Here's how the part is built. I have some questions about the finished solid (model axes, mm). A direction names the side the tool comes from. Coordinates: 2 decimals unless noted, no trailing zeros. Write each loop counter-clockwise with the first axis right and the second up, starting at its lowest first coordinate (ties: lowest second). Pieces come first, ordered by that corner, then holes. Notation, with made-up numbers: M -23,-0.5 L 19,-0.5 A12 ccw 19,17.5 Z; hole C -26.5,14 d8. An arc over 180 degrees is marked long. Use a Markdown table: item, result.
```python
from build123d import *

# Parameters (mm, degrees)
SKETCH1_W           = 60.96
SKETCH1_H           = 40.64
BOSS_EXTRUDE1_DEPTH = 17.78
SHELL1_T            = -2.54
SKETCH2_R           = 2.54
BOSS_EXTRUDE2_DEPTH = 17.78
SKETCH3_R           = 1.016
CUT_EXTRUDE2_DEPTH  = 7.62
SKETCH5_W           = 7.62
SKETCH5_H           = 3.81
CUT_EXTRUDE3_DEPTH  = 2.54
FILLET1_R           = 1.27
SKETCH6_W           = 40.64
SKETCH6_H           = 19.05
CUT_EXTRUDE4_DEPTH  = 2.54
FILLET3_R           = 2.54


with BuildPart() as part:
    # Sketch1 → Boss-Extrude1 (new body)
    with BuildSketch(Plane(origin=(0, 0, 0), x_dir=(1, 0, 0), z_dir=(0, 1, 0))):
        with Locations((30.48, 20.32)):
            Rectangle(SKETCH1_W, SKETCH1_H)
    extrude(amount=BOSS_EXTRUDE1_DEPTH)

    # Shell1
    shell1_openings = [part.faces().sort_by_distance(p)[0] for p in [
        (30.48, 17.78, -20.32),
    ]]
    offset(amount=SHELL1_T, openings=shell1_openings, kind=Kind.INTERSECTION)

    # Sketch2 → Boss-Extrude2 (add)
    with BuildSketch(Plane(origin=(0, 17.78, 0), x_dir=(1, 0, 0), z_dir=(0, 1, 0))):
        with Locations((2.54, 2.54)):
            Circle(SKETCH2_R)
        with Locations((58.42, 2.54)):
            Circle(SKETCH2_R)
        with Locations((58.42, 38.1)):
            Circle(SKETCH2_R)
        with Locations((2.54, 38.1)):
            Circle(SKETCH2_R)
    extrude(amount=-BOSS_EXTRUDE2_DEPTH)

    # Sketch3 → Cut-Extrude2 (cut)
    with BuildSketch(Plane(origin=(0, 17.78, 0), x_dir=(1, 0, 0), z_dir=(0, 1, 0))):
        with Locations(Location((2.525101816, 38.1, 0), (0, 0, 270))):
            Circle(SKETCH3_R)
        with Locations(Location((2.525101816, 2.54, 0), (0, 0, 270))):
            Circle(SKETCH3_R)
        with Locations(Location((58.42, 2.54, 0), (0, 0, 270))):
            Circle(SKETCH3_R)
        with Locations(Location((58.42, 38.1, 0), (0, 0, 270))):
            Circle(SKETCH3_R)
    extrude(amount=-CUT_EXTRUDE2_DEPTH, mode=Mode.SUBTRACT)

    # Sketch5 → Cut-Extrude3 (cut)
    with BuildSketch(Plane(origin=(60.96, 0, 0), x_dir=(0, 0, -1), z_dir=(1, 0, 0))):
        with Locations((15.24, 15.875)):
            Rectangle(SKETCH5_W, SKETCH5_H)
    extrude(amount=-CUT_EXTRUDE3_DEPTH, mode=Mode.SUBTRACT)

    # Fillet1
    fillet1_edges = [part.edges().sort_by_distance(p)[0] for p in [
        (59.69, 13.97, -19.05),
        (59.69, 13.97, -11.43),
    ]]
    fillet(fillet1_edges, radius=FILLET1_R)

    # Sketch6 → Cut-Extrude4 (cut)
    with BuildSketch(Plane.XZ):
        with Locations((35.56, -28.575)):
            Rectangle(SKETCH6_W, SKETCH6_H)
    extrude(amount=-CUT_EXTRUDE4_DEPTH, mode=Mode.SUBTRACT)

    # Fillet3
    fillet3_edges = [part.edges().sort_by_distance(p)[0] for p in [
        (30.48, 0, -40.64),
        (60.96, 0, -20.32),
        (30.48, 0, 0),
        (0, 0, -20.32),
        (0, 8.89, -40.64),
        (60.96, 8.89, -40.64),
        (60.96, 8.89, 0),
        (0, 8.89, 0),
    ]]
    fillet(fillet3_edges, radius=FILLET3_R - 0.0001)  # a hair under: the kernel refuses the full size


solid = part.part
```
1. Suppose I cut it at B-B on z = -31.5. Write out the boundary of the cut face in (x, y), and give its area (3 significant figures).
Answers follow:
| item | result |
|---|---|
| outline | M 0,2.54 A2.54 ccw 2.54,0 L 15.24,0 L 15.24,2.54 L 2.54,2.54 L 2.54,17.78 L 0,17.78 Z; M 55.88,0 L 58.42,0 A2.54 ccw 60.96,2.54 L 60.96,17.78 L 58.42,17.78 L 58.42,2.54 L 55.88,2.54 Z |
| area | 126 mm2 |
2. I need wall thicknesses on probe 1 along Z at (x, y) = (44.5, 16.25); probe 2 along X at (y, z) = (4, -19.5); probe 3 along Y at (x, z) = (31, -17.5). Which ranges of each line are inside material? Lowest first, please.
Answers follow:
| item | result |
|---|---|
| probe 1 | z = -40.64 to -38.1, -2.54 to 0 |
| probe 2 | x = 0 to 2.54, 58.42 to 60.96 |
| probe 3 | y = 0 to 2.54 |
3. Which directions (+Z, -Z, +X, -X, +Y, -Y) give clear straight access to the entire face, cutting with the end or side of a thin tool? Please do faces 5 (the face through (0, 10, -20)), 6 (the face through (60, 13.97, -15)), 7 (the face through (56.644, 10.267, -4.356)), 8 (the face through (30.871, 0.724, -0.764)), 9 (the face through (55.88, 1, -29)).
Answers follow:
| item | result |
|---|---|
| face 5 | +Z, -Z, -X, +Y, -Y |
| face 6 | +X, +Y |
| face 7 | +Y |
| face 8 | +Z, +X, -X, -Y |
| face 9 | +Y, -Y |
4. We'd pull the mould along X, two halves only. Please class faces 1 (the face through (0.764, 10.267, -0.724)), 2 (the face through (59.672, 14.352, -18.688)), 3 (the face through (3, 10.16, -38)), 4 (the face through (30, 10, -2.54)): +X half, -X half, draft (parallel to the pull), parting line (faces both ways), or undercut.
Answers follow:
| item | result |
|---|---|
| face 1 | -X half |
| face 2 | draft |
| face 3 | undercut |
| face 4 | undercut |
5. Suppose I cut it at D-D on x = 8.5. Write out the boundary of the cut face in (y, z).
Answers follow:
| item | result |
|---|---|
| outline | M 0,-38.1 A2.54 ccw 2.54,-40.64 L 17.78,-40.64 L 17.78,-38.1 L 2.54,-38.1 L 2.54,-2.54 L 17.78,-2.54 L 17.78,0 L 2.54,0 A2.54 ccw 0,-2.54 Z |
6. Suppose I cut it at C-C on z = -15. Write out the boundary of the cut face in (x, y), and give its area (3 significant figures).
Answers follow:
| item | result |
|---|---|
| outline | M 0,2.54 A2.54 ccw 2.54,0 L 58.42,0 A2.54 ccw 60.96,2.54 L 60.96,13.97 L 58.42,13.97 L 58.42,2.54 L 2.54,2.54 L 2.54,17.78 L 0,17.78 Z |
| area | 220 mm2 |
7. Will these pins go through, and if not, where does the flat tip stop? pin 1 Ø1.3 at (x, y) = (60.5, 17) entering from -Z; pin 2 Ø2.5 at (x, z) = (2.53, -38.1) entering from +Y; pin 3 Ø1.3 at (y, z) = (1.5, -33) entering from -X; pin 4 Ø1.2 at (x, z) = (58.42, -2.54) entering from +Y.
Answers follow:
| item | result |
|---|---|
| pin 1 | stops at z = -40.2 |
| pin 2 | stops at y = 17.78 |
| pin 3 | stops at x = 0.03 |
| pin 4 | stops at y = 10.16 |
